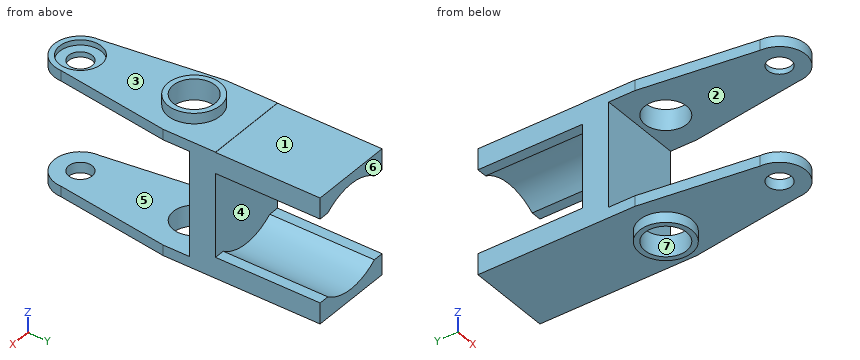
from build123d import *

# Parameters (mm, degrees)
SKETCH_4_R                   = 4
EXTRUDE_1_DEPTH              = 24
HOLE_WIZARD_M4_1_D           = 4.5
HOLE_WIZARD_M4_1_CBORE_D     = 8
HOLE_WIZARD_M4_1_CBORE_DEPTH = 1
EXTRUDE_2_DEPTH              = 2
EXTRUDE_2_DEPTH_BACK         = 26
SKETCH_7_R                   = 5
SKETCH_7_R_2                 = 4
EXTRUDE_3_DEPTH              = 20
CUT_EXTRUDE_1_DEPTH          = 20


with BuildPart() as part:
    # 草图4 → 凸台-拉伸1 (new body)
    with BuildSketch(Plane.XY):
        with BuildLine():
            Line((-8, 0), (-5, -21.75))
            ThreePointArc((-5, -21.75), (0, -26.75), (5, -21.75))
            Line((5, -21.75), (8, 0))
            Line((8, 0), (8, 10))
            Line((8, 10), (5, 10))
            Line((5, 10), (-5, 10))
            Line((-5, 10), (-8, 10))
            Line((-8, 10), (-8, 0))
        make_face()
        Circle(SKETCH_4_R, mode=Mode.SUBTRACT)
    extrude(amount=EXTRUDE_1_DEPTH)

    # M4 六角凹头盖的柱孔1 (through all)
    with Locations(Plane(origin=(0, -21.75, 24), x_dir=(1, 0, 0), z_dir=(0, 0, 1))):
        with Locations((0, 0)):
            CounterBoreHole(HOLE_WIZARD_M4_1_D / 2, HOLE_WIZARD_M4_1_CBORE_D / 2, HOLE_WIZARD_M4_1_CBORE_DEPTH)

    # 草图7 → 凸台-拉伸2 (add, two sides: drawn at the far end of the back side and taken through both)
    with BuildSketch(Plane.XY.offset(24).offset(-EXTRUDE_2_DEPTH_BACK)):
        Circle(SKETCH_7_R)
        Circle(SKETCH_7_R_2, mode=Mode.SUBTRACT)
    extrude(amount=EXTRUDE_2_DEPTH + EXTRUDE_2_DEPTH_BACK)

    # 草图8 → 凸台-拉伸3 (add)
    with BuildSketch(Plane(origin=(0, 10, 0), x_dir=(1, 0, 0), z_dir=(0, 1, 0))):
        with BuildLine():
            Line((-8, 0), (8, 0))
            Line((8, 0), (8, -4))
            Line((8, -4), (6.008972597, -4))
            ThreePointArc((6.008972597, -4), (0, -1.989201574), (-6.008972597, -4))
            Line((-6.008972597, -4), (-8, -4))
            Line((-8, -4), (-8, 0))
        make_face()
        with BuildLine():
            Line((8, -23.946124164), (8, -19.946124164))
            Line((8, -19.946124164), (6.008972597, -19.946124164))
            ThreePointArc((6.008972597, -19.946124164), (0, -21.956922589), (-6.008972597, -19.946124164))
            Line((-6.008972597, -19.946124164), (-8, -19.946124164))
            Line((-8, -19.946124164), (-8, -23.946124164))
            Line((-8, -23.946124164), (8, -23.946124164))
        make_face()
    extrude(amount=EXTRUDE_3_DEPTH)

    # 草图9 → 切除-拉伸1 (cut)
    with BuildSketch(Plane.ZY.offset(8)):
        Polygon((2, -27), (2, 0), (2, 5), (22, 5), (22, -27), align=None)
    extrude(amount=-CUT_EXTRUDE_1_DEPTH, mode=Mode.SUBTRACT)


solid = part.part
The listing builds one solid part. Answer for the finished solid, in the listing's coordinates (mm). Face numbers are marked on the shaded views. A direction names the side the tool comes from. Give positions to 0.01 mm unless a question says otherwise; leave off trailing zeros. Write each loop counter-clockwise with the first axis right and the second up, starting at its lowest first coordinate (ties: lowest second). Pieces come first, ordered by that corner, then holes.
Item 1: Flat-ended cylindrical pins translate along their axes: P1, Ø1.6, axis at x = -7.5, y = 21, coming from the +Z side; P2, Ø5, axis at x = 2.5, z = 8, coming from the -Y side; P3, Ø2.5, axis at x = 0, y = -21.75, coming from the +Z side (1 decimal); P4, Ø5, axis at x = 0, y = -17, coming from the +Z side. Find the tip coordinate at first contact, or state that the pin passes through.
Item 2: Determine the mould class of the marked faces 5, 6 and 7 for opening direction Y: released by +Y, released by -Y, zero draft, split by the parting line, or undercut.
Item 3: Section D-D, the plane z = 14 is taken. Write down the section's boundary in (x, y), plus the area to 3 significant figures.
Item 4: Find the intervals of material crossed by line 1 along Y through (x, z) = (0, 23.6); line 2 along Y through (x, z) = (0, 22.6); line 3 along Z through (x, y) = (-7, 0), in increasing order.
Item 5: Section B-B, the plane y = -12 is taken. Write down the section's boundary in (x, z).
Item 6: Section C-C, the plane x = 0 is taken. Count the separate pieces of the cut face and the enclosed holes in it, plus the area to 3 significant figures.
Item 7: Which of the six approach directions +Z, -Z, +X, -X, +Y, -Y give full straight-line access (tool end or side, diameter ignored) to the marked faces 1, 2, 3 and 4?
Item 8: Section A-A, the plane y = 1.5 is taken. Write down the section's boundary in (x, z), plus the area to 3 significant figures.
Completed:
1. P1: stops at z = 23.95
1. P2: stops at y = 5
1. P3: passes through
1. P4: stops at z = 24
2. face 5: zero draft
2. face 6: released by +Y
2. face 7: undercut
3. outline: (-8, 5) - (8, 5) - (8, 10) - (-8, 10) - close
3. area: 80.0 mm2
4. line 1: y = -26.75 to -25.75, -17.75 to -4, 4 to 30
4. line 2: y = -26.75 to -24, -19.5 to -4, 4 to 30
4. line 3: z = 0 to 2, 22 to 24
5. outline: (-6.34, 0) - (6.34, 0) - (6.34, 2) - (-6.34, 2) - close; (-6.34, 22) - (6.34, 22) - (6.34, 24) - (-6.34, 24) - close
6. separate pieces: 5
6. enclosed holes: 0
6. area: 281 mm2
7. face 1: +Z, +X, -X, +Y
7. face 2: +X, -X, -Y
7. face 3: +Z
7. face 4: +Y
8. outline: (-8, 0) - (-4.77, 0) - (-4.77, -2) - (-3.71, -2) - (-3.71, 2) - (-8, 2) - close; (-8, 22) - (-3.71, 22) - (-3.71, 26) - (-4.77, 26) - (-4.77, 24) - (-8, 24) - close; (3.71, -2) - (4.77, -2) - (4.77, 0) - (8, 0) - (8, 2) - (3.71, 2) - close; (3.71, 22) - (8, 22) - (8, 24) - (4.77, 24) - (4.77, 26) - (3.71, 26) - close
8. area: 42.8 mm2
